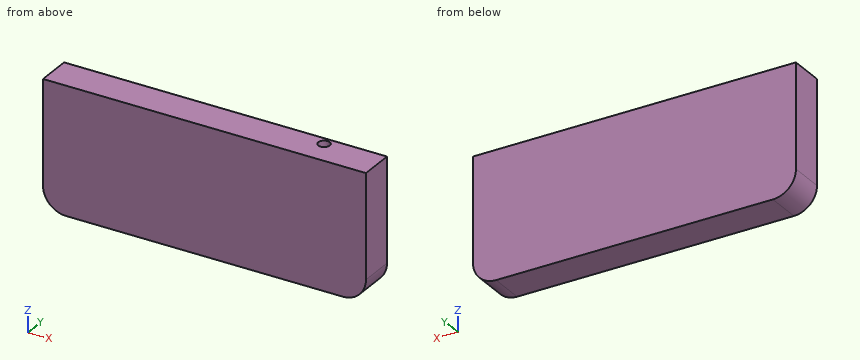
from build123d import *

# Parameters (mm, degrees)
BOSS_EXTRU_1_DEPTH      = 30
ESQUISSE2_R             = 5
ENL_V_MAT_EXTRU_1_DEPTH = 58


with BuildPart() as part:
    # Esquisse1 → Boss.-Extru.1 (new body)
    with BuildSketch(Plane(origin=(0, 0, 0), x_dir=(1, 0, 0), z_dir=(0, 1, 0))):
        with BuildLine():
            Line((0, 0), (280, 0))
            Line((280, 0), (280, 90))
            ThreePointArc((280, 90), (274.142135624, 104.142135624), (260, 110))
            Line((260, 110), (20, 110))
            ThreePointArc((20, 110), (5.857864376, 104.142135624), (0, 90))
            Line((0, 90), (0, 0))
        make_face()
    extrude(amount=-BOSS_EXTRU_1_DEPTH)

    # Esquisse2 → Enlèv. mat.-Extru.1 (cut)
    with BuildSketch(Plane.XY):
        with Locations((230, -7.5)):
            Circle(ESQUISSE2_R)
    extrude(amount=-ENL_V_MAT_EXTRU_1_DEPTH, mode=Mode.SUBTRACT)


solid = part.part
Check sheet for the modelled part. Datum: model origin and axes. Units: mm. Round coordinates to 2 decimals unless told otherwise and drop trailing zeros. Loops run counter-clockwise (first coordinate to the right, second up) from the corner with the lowest first, then second, coordinate; pieces in that order, holes last. Notation, with made-up numbers: (48, -32.5) - (101, -32.5) arc R14 ccw to (101, -24.5) - close; hole circle Ø9 at (-35.5, 13.5). An arc over 180 degrees is marked (long way). Answer as CSV lines item,"result". Start each with the question number.
Item 1: Section check B-B (x = 230). Record the boundary of the cut face in (y, z).
Item 2: Depth check by flat-ended pin: P1, Ø1.5, axis at y = -24, z = -97, coming from the -X side; P2, Ø3, axis at x = 231.5, y = -6.5, coming from the +Z side; P3, Ø2, axis at x = 68, y = -18, coming from the +Z side. Enter the tip coordinate at first touch or a pass-through.
Item 3: Scan lines: line 1 (Y direction, x = 230, z = -32); line 2 (X direction, y = -10.5, z = -47); line 3 (X direction, y = -3, z = -44). Record each from-to range of solid material in increasing order. Write a range as [from, to].
Item 4: Section check A-A (y = -7.5). Record the boundary of the cut face in (x, z), and give its area (3 significant figures).
Report:
1,outline,"(-30, -110) - (0, -110) - (0, 0) - (-2.5, 0) - (-2.5, -58) - (-12.5, -58) - (-12.5, 0) - (-30, 0) - close"
2,P1,"stops at x = 1"
2,P2,"stops at z = -58"
2,P3,"stops at z = 0"
3,line 1,"y = [-30, -12.5], [-2.5, 0]"
3,line 2,"x = [0, 226], [234, 280]"
3,line 3,"x = [0, 227.82], [232.18, 280]"
4,outline,"(0, -90) arc R20 ccw to (20, -110) - (260, -110) arc R20 ccw to (280, -90) - (280, 0) - (235, 0) - (235, -58) - (225, -58) - (225, 0) - (0, 0) - close"
4,area,"30,000 mm2"
